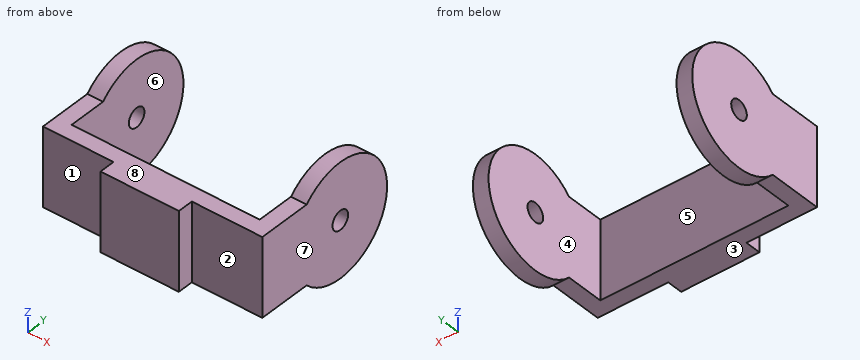
from build123d import *

# Parameters (mm, degrees)
SKETCH1_W           = 35
SKETCH1_H           = 25
BOSS_EXTRUDE1_DEPTH = 5
SKETCH7_R           = 18
SKETCH7_R_2         = 3
BOSS_EXTRUDE2_DEPTH = 5
SKETCH8_W           = 25
SKETCH8_H           = 25
BOSS_EXTRUDE3_DEPTH = 5


with BuildPart() as part:
    # Sketch1 → Boss-Extrude1 (new body)
    with BuildSketch(Plane(origin=(0, 0, 0), x_dir=(1, 0, 0), z_dir=(0, 1, 0))):
        with Locations((17.5, 0)):
            Rectangle(SKETCH1_W, SKETCH1_H)
    boss_extrude1 = extrude(amount=BOSS_EXTRUDE1_DEPTH)

    # Sketch7 → Boss-Extrude2 (add)
    # profile 1 of 2: a face of its own
    with BuildSketch(Plane(origin=(35, 0, 0), x_dir=(0, 0, -1), z_dir=(1, 0, 0))):
        with Locations((0, 30)):
            Circle(SKETCH7_R)
        with Locations((0, 30)):
            Circle(SKETCH7_R_2, mode=Mode.SUBTRACT)
    # profile 2 of 2: a face of its own
    with BuildSketch(Plane(origin=(35, 0, 0), x_dir=(0, 0, -1), z_dir=(1, 0, 0))):
        with BuildLine():
            Line((-12.5, 17.048166153), (-12.5, 5))
            Line((-12.5, 5), (12.5, 5))
            Line((12.5, 5), (12.5, 17.048166153))
            ThreePointArc((12.5, 17.048166153), (0, 12), (-12.5, 17.048166153))
        make_face()
    boss_extrude2 = extrude(amount=-BOSS_EXTRUDE2_DEPTH)

    # Mirror1: Boss-Extrude1, Boss-Extrude2 across plane
    add(boss_extrude1.mirror(Plane(origin=(0, 5, -12.5), x_dir=(0, 0, 1), z_dir=(1, 0, 0))))
    add(boss_extrude2.mirror(Plane(origin=(0, 5, -12.5), x_dir=(0, 0, 1), z_dir=(1, 0, 0))))

    # Sketch8 → Boss-Extrude3 (add)
    with BuildSketch(Plane.XZ):
        Rectangle(SKETCH8_W, SKETCH8_H)
    extrude(amount=BOSS_EXTRUDE3_DEPTH)


solid = part.part
The listing builds one solid part. Answer for the finished solid, in the listing's coordinates (mm). Face numbers are marked on the shaded views. A direction names the side the tool comes from. Give positions to 0.01 mm unless a question says otherwise; leave off trailing zeros. Loops run counter-clockwise (first coordinate to the right, second up) from the corner with the lowest first, then second, coordinate; pieces in that order, holes last. Notation, with made-up numbers: M -31,28 L -12,28 A17 cw -12,52 Z; hole C -2,75 d10. An arc over 180 degrees is marked long. Answer as CSV lines item,"result".
Item 1: Which of the six approach directions +Z, -Z, +X, -X, +Y, -Y give full straight-line access (tool end or side, diameter ignored) to the marked faces 1, 2, 3 and 4?
Values follow:
face 1,"+Z, -Z, -X, -Y"
face 2,"+Z, -Z, +X, -Y"
face 3,"-Z, +X, -X, -Y"
face 4,"+Z, -Z, +Y"
Item 2: The part is cut by section D-D (z = 14.5). Give the vertices of the cut face in (x, y), and give its area (3 significant figures).
Values follow:
outline,"M -35,19.33 L -30,19.33 L -30,40.67 L -35,40.67 Z; M 30,19.33 L 35,19.33 L 35,40.67 L 30,40.67 Z"
area,"213 mm^2"
Item 3: The part is cut by section A-A (y = 30). Give the vertices of the cut face in (x, z), and give its area (3 significant figures).
Values follow:
outline,"M -35,-18 L -30,-18 L -30,-3 L -35,-3 Z; M -35,3 L -30,3 L -30,18 L -35,18 Z; M 30,-18 L 35,-18 L 35,-3 L 30,-3 Z; M 30,3 L 35,3 L 35,18 L 30,18 Z"
area,"300 mm^2"
Item 4: Straight lines are drawn through the part: line 1 along X through (y, z) = (34.5, -6.5); line 2 along Y through (x, z) = (32.8, 0); line 3 along Y through (x, z) = (1, 1.5). For each, find the intervals that lie inside material, in ascending order. Write a range as [from, to].
Values follow:
line 1,"x = [-35, -30], [30, 35]"
line 2,"y = [0, 27], [33, 48]"
line 3,"y = [-5, 5]"
Item 5: Given pin 1 Ø7.5 at (x, z) = (11.5, -6) entering from +Y; pin 2 Ø18 at (x, z) = (-26, -4.5) entering from -Y; pin 3 Ø3 at (x, y) = (14, 1) entering from +Z, each flat-ended and moving along its own axis, determine where each tip first touches the part or whether it passes through.
Values follow:
pin 1,"stops at y = 5"
pin 2,"stops at y = 0"
pin 3,"stops at z = 12.5"
Item 6: The mould has two halves that part along X. Classify the marked faces 5, 6, 7 and 8: released by +X, released by -X, zero draft, split by the parting line, or undercut.
Values follow:
face 5,"undercut"
face 6,"undercut"
face 7,"released by +X"
face 8,"zero draft"
Item 7: The part is cut by section B-B (z = 0). Give the vertices of the cut face in (x, y).
Values follow:
outline,"M -35,0 L -12.5,0 L -12.5,-5 L 12.5,-5 L 12.5,0 L 35,0 L 35,27 L 30,27 L 30,5 L -30,5 L -30,27 L -35,27 Z; M -35,33 L -30,33 L -30,48 L -35,48 Z; M 30,33 L 35,33 L 35,48 L 30,48 Z"
Item 8: The part is cut by section C-C (y = 13). Give the vertices of the cut face in (x, z).
Values follow:
outline,"M -35,-12.5 L -30,-12.5 L -30,12.5 L -35,12.5 Z; M 30,-12.5 L 35,-12.5 L 35,12.5 L 30,12.5 Z"
